Here's the drawing with two shaded views (mm, measured from the low corner). I have some questions. A direction names the side the tool comes from. Give positions to 0.01 mm unless a question says otherwise; leave off trailing zeros. Write each loop counter-clockwise with the first axis right and the second up, starting at its lowest first coordinate (ties: lowest second). Pieces come first, ordered by that corner, then holes. Notation, with made-up numbers: (61.5, -15) - (95.5, -15) arc R19 cw to (95.5, 12) - close; hole circle Ø5 at (47, 46). An arc over 180 degrees is marked (long way). Answer as a JSON object with one key per item and string values. Group by question number.
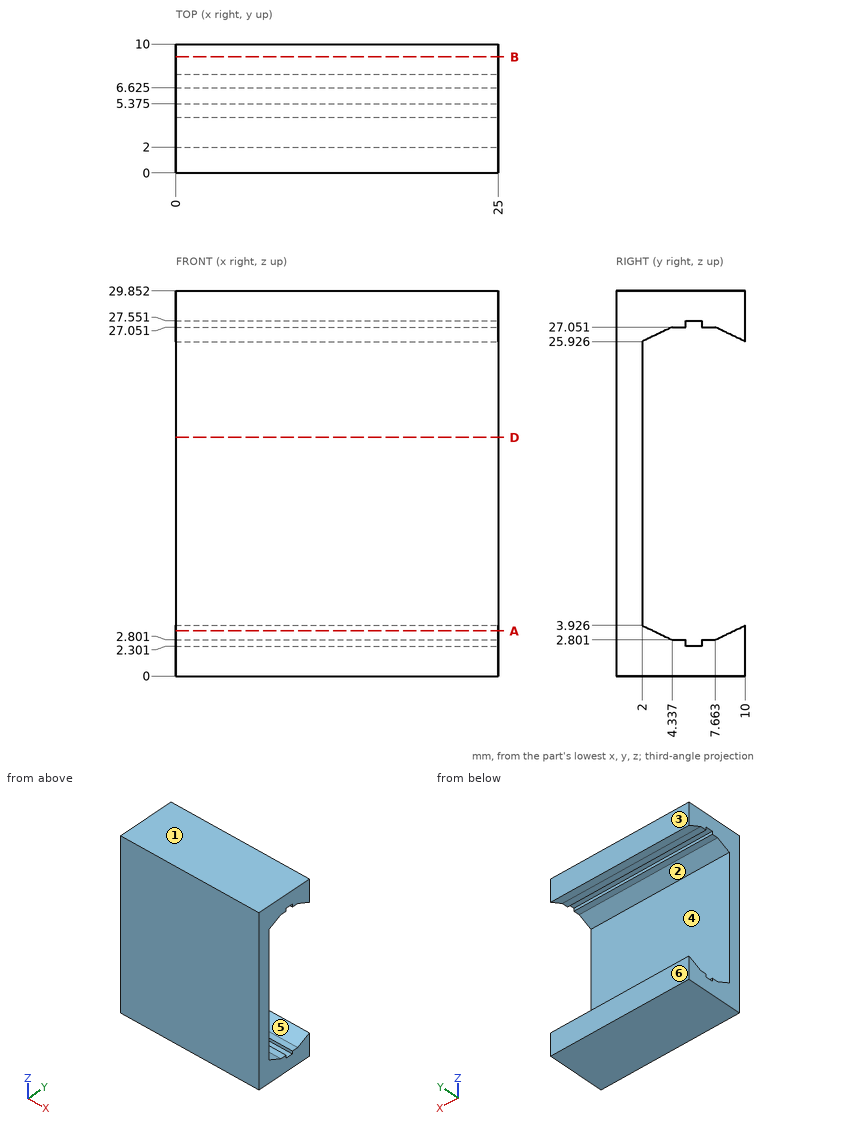
(1) I want a section at B-B, the plane y = 9. Please give me the cut outline in (x, z) (1 decimal), and give its area (3 significant figures).
(2) I want a section at A-A, the plane z = 3.5. Please give me the cut outline in (x, y) (1 decimal).
(3) I want a section at D-D, the plane z = 18.5. Please give me the cut outline in (x, y).
(4) Will this pin go through, and if not, where does the flat tip stop? P1, Ø1, axis at x = 21, z = 14.5, coming from the +Y side.
(5) For the marked faces 4, 5 and 6, which set-ups out of +Z, -Z, +X, -X, +Y, -Y let a thin tool reach every point of the face, with its end or its side?
(6) If we mould it in two halves opening along Z, with no side actions, what happens to the marked faces 1, 2 and 3? For each: +Z half, -Z half, draft (parallel to the pull), parting line (faces both ways), or undercut.
(7) I need wall thicknesses on L1, parallel to Z at x = 21.75, y = 6.25; L2, parallel to Y at x = 10, z = 24; L3, parallel to Y at x = 6.5, z = 3 (1 decimal). Which ranges of each line are inside material? Lowest first, please.
Entries:
{
 "1": {"outline": "(0, 0) - (25, 0) - (25, 3.4) - (0, 3.4) - close; (0, 26.4) - (25, 26.4) - (25, 29.9) - (0, 29.9) - close", "area": "172 mm^2"},
 "2": {"outline": "(0, 0) - (25, 0) - (25, 2.9) - (0, 2.9) - close; (0, 9.1) - (25, 9.1) - (25, 10) - (0, 10) - close"},
 "3": {"outline": "(0, 0) - (25, 0) - (25, 2) - (0, 2) - close"},
 "4": {"P1": "y = 2"},
 "5": {"face 4": "+X, -X, +Y", "face 5": "+X, -X", "face 6": "+Z, -Z, +X, -X, +Y"},
 "6": {"face 1": "+Z half", "face 2": "undercut", "face 3": "draft"},
 "7": {"L1": "0 to 2.3, 27.55 to 29.85", "L2": "0 to 2", "L3": "0 to 3.9, 8.1 to 10"}
}
